```python
from build123d import *

# Parameters (mm, degrees)
F0_R           = 12.75
F1_DEPTH       = 4
F3_D           = 4.7
F3_CSINK_D     = 14
F3_CSINK_ANGLE = 110
F4_R           = 1.75
F5_DEPTH       = 4.001


with BuildPart() as f1:
    # F0 (on Top) → F1 (new body)
    with BuildSketch(Plane.XY):
        Circle(F0_R)
    extrude(amount=F1_DEPTH)

    # F3 (through all)
    with Locations(Plane.XY.offset(4)):
        with Locations((0, 0)):
            CounterSinkHole(F3_D / 2, F3_CSINK_D / 2, counter_sink_angle=F3_CSINK_ANGLE)

    # F4 (on face) → F5 (cut, through all)
    with BuildSketch(Plane.XY.offset(4)):
        with Locations((0, -9.7)):
            Circle(F4_R)
        with Locations((0, 9.7)):
            Circle(F4_R)
    extrude(amount=-F5_DEPTH, mode=Mode.SUBTRACT)


solid = f1.part
```
Model file for the job. Use its own axes, mm. Give positions to 0.01 mm unless a question says otherwise; leave off trailing zeros. Loops run counter-clockwise (first coordinate to the right, second up) from the corner with the lowest first, then second, coordinate; pieces in that order, holes last. Notation, with made-up numbers: (18.25, -13) -> (38.25, -13) arc R33 ccw to (38.25, 24) -> close; hole circle Ø5 at (-12.75, 87). An arc over 180 degrees is marked (long way). Use CSV: the item, a comma, the result in double quotes. Start each with the question number.
1) Slice it at D-D on x = 10. Give the cut face in (y, z), plus the area to 3 significant figures.
2) Slice it at A-A on y = 0. Give the cut face in (x, z).
3) Flat gauge pins, fed straight in: pin 1 Ø2 at (y, z) = (6.5, 1) entering from -X; pin 2 Ø2 at (x, y) = (1, 2.5) entering from +Z; pin 3 Ø2 at (y, z) = (-3, 1) entering from +X. Where does each tip first touch, or does it go through?
4) Wall check: line 1 (Y direction, x = 0, z = 0.6); line 2 (Y direction, x = 0, z = 0.95); line 3 (X direction, y = 3.5, z = 3.85). Give the ranges that are in metal, low to high.
5) Mould opens along Y. For faces 1 (the cylindrical face through (-2.764, -12.447, 1.972)), 2 (the flat face through (3, 0, 0)), 3 (the cylindrical face through (-0.228, 11.435, 2.028)) say: released by +Y, released by -Y, zero draft, split by the parting line, or undercut.
6) Slice it at B-B on y = 9.25. Give the cut face in (x, z).
7) Slice it at C-C on z = 1.6. Give the cut face in (x, y).
Computed values:
1,outline,"(-7.91, 0) -> (7.91, 0) -> (7.91, 4) -> (-7.91, 4) -> close"
1,area,"63.3 mm^2"
2,outline,"(-12.75, 0) -> (-2.35, 0) -> (-2.35, 0.74) -> (-7, 4) -> (-12.75, 4) -> close; (2.35, 0) -> (12.75, 0) -> (12.75, 4) -> (7, 4) -> (2.35, 0.74) -> close"
3,pin 1,"stops at x = -11.5"
3,pin 2,"stops at z = 1.68"
3,pin 3,"stops at x = 12.59"
4,line 1,"y = -12.75 to -11.45, -7.95 to -2.35, 2.35 to 7.95, 11.45 to 12.75"
4,line 2,"y = -12.75 to -11.45, -7.95 to -2.64, 2.64 to 7.95, 11.45 to 12.75"
4,line 3,"x = -12.26 to -5.81, 5.81 to 12.26"
5,face 1,"split by the parting line"
5,face 2,"zero draft"
5,face 3,"undercut"
6,outline,"(-8.77, 0) -> (-1.69, 0) -> (-1.69, 4) -> (-8.77, 4) -> close; (1.69, 0) -> (8.77, 0) -> (8.77, 4) -> (1.69, 4) -> close"
7,outline,"circle Ø25.5 at (0, 0); hole circle Ø7.14 at (0, 0); hole circle Ø3.5 at (0, -9.7); hole circle Ø3.5 at (0, 9.7)"
